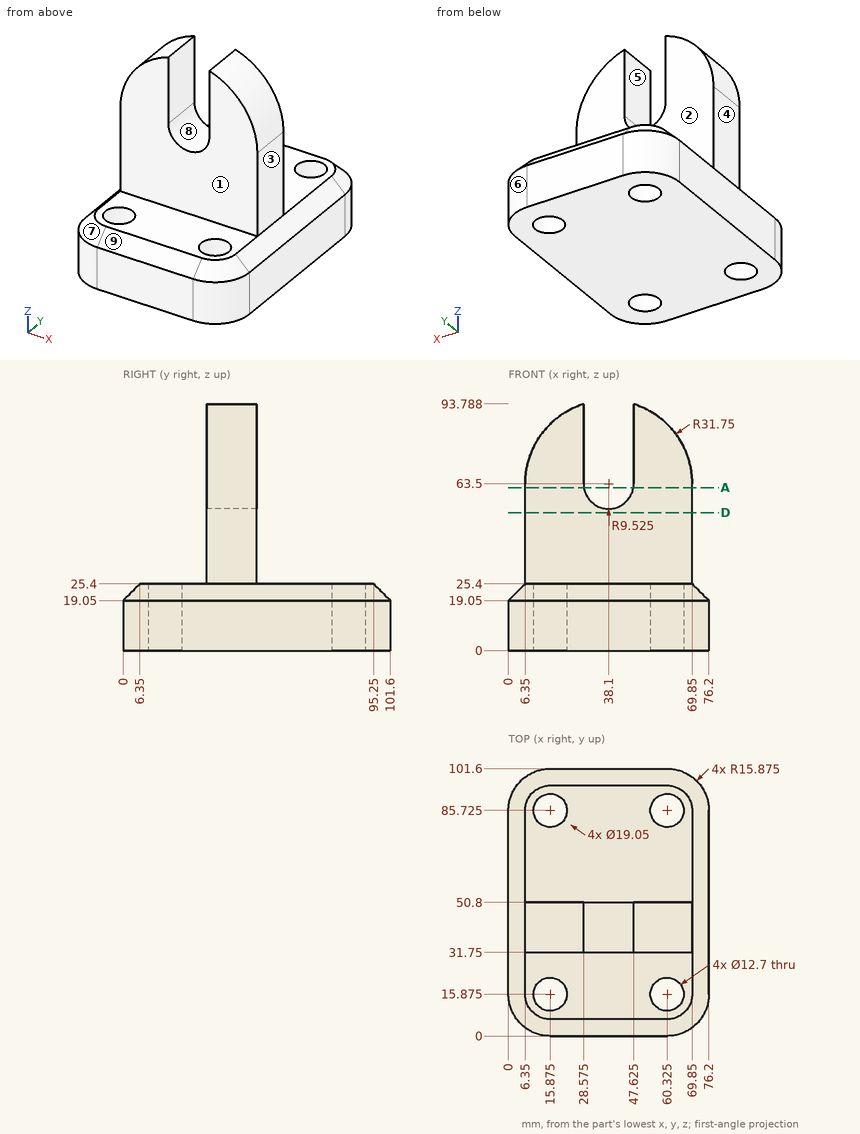
Study the drawing (mm; zero at the part's minimum x, y, z) and answer. A direction names the side the tool comes from. Give positions to 0.01 mm unless a question says otherwise; leave off trailing zeros. Loops run counter-clockwise (first coordinate to the right, second up) from the corner with the lowest first, then second, coordinate; pieces in that order, holes last. Notation, with made-up numbers: (85.25, 39.25) -> (141.25, 39.25) arc R23 ccw to (141.25, 57.25) -> close; hole circle Ø9 at (-32.75, -25.5). An arc over 180 degrees is marked (long way). Write item = value, one per line. Start each with the question number.
(1) Find section A-A on z = 62. Give the vertices of the cut face in (x, y), and give its area (3 significant figures).
(2) Find the intervals of material crossed by probe 1 along Y at (x, z) = (64.5, 64.5); probe 2 along Z at (x, y) = (48.5, 64.5); probe 3 along X at (y, z) = (48, 47.5), in increasing order. Write a range as from..to.
(3) Find section D-D on z = 52.5. Give the vertices of the cut face in (x, y).
(4) Given pin 1 Ø14.5 at (x, y) = (60.325, 15.875) entering from +Z; pin 2 Ø7.5 at (x, y) = (15.875, 85.725) entering from -Z; pin 3 Ø9.5 at (y, z) = (42, 51.5) entering from -X; pin 4 Ø1 at (x, z) = (61.5, 14.5) entering from -Y, each flat-ended and moving along its own axis, determine where each tip first touches the part or whether it passes through.
(5) The mould has two halves that part along X. Classify the marked faces 6, 7, 8 and 9: +X half, -X half, draft (parallel to the pull), parting line (faces both ways), or undercut.
(6) Which of the six approach directions +Z, -Z, +X, -X, +Y, -Y give full straight-line access (tool end or side, diameter ignored) to the marked faces 1, 2, 3, 4 and 5?
From the geometry:
q1.outline = (6.35, 31.75) -> (28.69, 31.75) -> (28.69, 50.8) -> (6.35, 50.8) -> close; (47.51, 31.75) -> (69.85, 31.75) -> (69.85, 50.8) -> (47.51, 50.8) -> close
q1.area = 851 mm^2
q2.probe_1 = 31.75..50.8
q2.probe_2 = 0..25.4
q2.probe_3 = 6.35..69.85
q3.outline = (6.35, 31.75) -> (69.85, 31.75) -> (69.85, 50.8) -> (6.35, 50.8) -> close
q4.pin_1 = 25.4
q4.pin_2 = through
q4.pin_3 = 6.35
q4.pin_4 = 0.01
q5.face_6 = +X half
q5.face_7 = -X half
q5.face_8 = undercut
q5.face_9 = draft
q6.face_1 = +Z, +X, -X, -Y
q6.face_2 = +Z, +X, -X, +Y
q6.face_3 = +Z, +X, +Y, -Y
q6.face_4 = +Z, -X, +Y, -Y
q6.face_5 = +Z, +Y, -Y
